```python
from build123d import *

# Parameters (mm, degrees)
SKETCH1_R               = 22.5
BOSS_EXTRUDE1_DEPTH     = 15
SKETCH2_R               = 2.75
CUT_EXTRUDE1_DEPTH      = 36.178118199
SKETCH5_R               = 8.1
CUT_EXTRUDE2_DEPTH      = 5.5
SKETCH6_R               = 5.25
CUT_EXTRUDE3_DEPTH      = 5.5
CIRPATTERN1_COUNT       = 8
SKETCH29_R              = 22.5
SKETCH29_R_2            = 12.5
CUT_EXTRUDE_THIN1_DEPTH = 2


with BuildPart() as part:
    # Sketch1 → Boss-Extrude1 (new body)
    with BuildSketch(Plane(origin=(0, 0, 0), x_dir=(0, 0, -1), z_dir=(1, 0, 0))):
        Circle(SKETCH1_R)
    extrude(amount=-BOSS_EXTRUDE1_DEPTH)

    # Sketch2 → Cut-Extrude1 (cut, through all)
    with BuildSketch(Plane(origin=(0, 0, 0), x_dir=(0, 0, -1), z_dir=(1, 0, 0))):
        Circle(SKETCH2_R)
    extrude(amount=-CUT_EXTRUDE1_DEPTH, mode=Mode.SUBTRACT)

    # Sketch5 → Cut-Extrude2 (cut)
    with BuildSketch(Plane.ZY.offset(15)):
        Circle(SKETCH5_R)
    extrude(amount=-CUT_EXTRUDE2_DEPTH, mode=Mode.SUBTRACT)

    # Sketch6 → Cut-Extrude3 (cut)
    with BuildSketch(Plane.XY.offset(22.5)):
        with Locations((-9, 0)):
            Circle(SKETCH6_R)
    cut_extrude3 = extrude(amount=-CUT_EXTRUDE3_DEPTH, mode=Mode.SUBTRACT)

    # CirPattern1: Cut-Extrude3 ×8 about axis
    cirpattern1_axis = Axis((0, 0, 0), (1, 0, 0))
    for i in range(1, CIRPATTERN1_COUNT):
        add(cut_extrude3.rotate(cirpattern1_axis, i * 360 / CIRPATTERN1_COUNT), mode=Mode.SUBTRACT)

    # Sketch29 → Cut-Extrude-Thin1 (cut)
    with BuildSketch(Plane(origin=(0, 0, 0), x_dir=(0, 0, -1), z_dir=(1, 0, 0))):
        Circle(SKETCH29_R)
        Circle(SKETCH29_R_2, mode=Mode.SUBTRACT)
    extrude(amount=-CUT_EXTRUDE_THIN1_DEPTH, mode=Mode.SUBTRACT)


solid = part.part
```
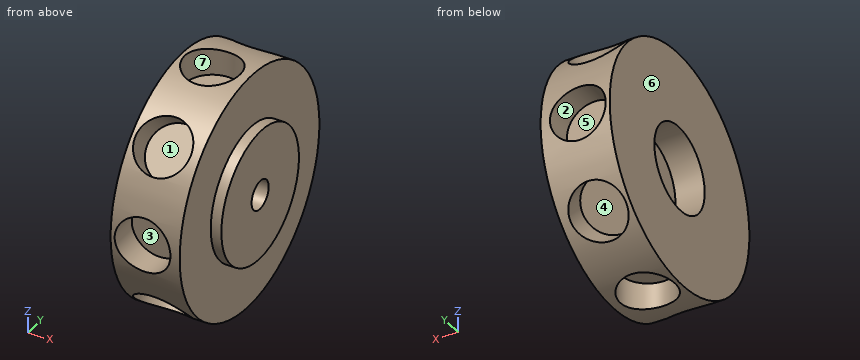
Check sheet for the modelled part. Datum: model origin and axes. Units: mm. Face numbers are marked on the shaded views. A direction names the side the tool comes from. Round coordinates to 2 decimals unless told otherwise and drop trailing zeros. Loops run counter-clockwise (first coordinate to the right, second up) from the corner with the lowest first, then second, coordinate; pieces in that order, holes last. Notation, with made-up numbers: (26.25, -21.5) -> (52.25, -21.5) arc R24 cw to (52.25, 3.5) -> close; hole circle Ø5 at (43.25, 43). An arc over 180 degrees is marked (long way). Write item = value, one per line. Start each with the question number.
1) Release check for a two-part mould opening along Y. For the marked faces 4, 5, 6 and 7 record: released by +Y, released by -Y, zero draft, split by the parting line, or undercut.
2) Sectioned sample at D-D, the plane y = 6.5. Record the cut outline in (x, z), plus the area to 3 significant figures.
3) Sectioned sample at A-A, the plane z = 0. Record the cut outline in (x, y), plus the area to 3 significant figures.
4) Set-up check for the marked faces 1, 2 and 3: record each of +Z, -Z, +X, -X, +Y, -Y from which the full face is reachable in a straight line by a thin tool's end or side.
5) Gauge pin test, flat ends, axial feed: pin 1 Ø5 at (x, y) = (-10, 1) entering from +Z; pin 2 Ø1 at (y, z) = (17, 3) entering from +X; pin 3 Ø5 at (x, y) = (-11.5, -14.5) entering from -Z. Record the tip position at first contact, or that the pin passes through.
6) Thickness scan on probe 1 along Z at (x, y) = (-6.5, -11.5); probe 2 along X at (y, z) = (0, -20); probe 3 along Y at (x, z) = (-5.25, 0). Record the ranges inside material, lowest first.
Results are:
q1.face_4 = undercut
q1.face_5 = released by +Y
q1.face_6 = zero draft
q1.face_7 = undercut
q2.outline = (-15, -21.54) -> (-2, -21.54) -> (-2, -10.68) -> (0, -10.68) -> (0, 10.68) -> (-2, 10.68) -> (-2, 21.54) -> (-15, 21.54) -> (-15, 4.83) -> (-9.5, 4.83) -> (-9.5, -4.83) -> (-15, -4.83) -> close
q2.area = 550 mm^2
q3.outline = (-15, -22.5) -> (-14.25, -22.5) -> (-14.25, -17) -> (-3.75, -17) -> (-3.75, -22.5) -> (-2, -22.5) -> (-2, -12.5) -> (0, -12.5) -> (0, -2.75) -> (-9.5, -2.75) -> (-9.5, -8.1) -> (-15, -8.1) -> close; (-15, 8.1) -> (-9.5, 8.1) -> (-9.5, 2.75) -> (0, 2.75) -> (0, 12.5) -> (-2, 12.5) -> (-2, 22.5) -> (-3.75, 22.5) -> (-3.75, 17) -> (-14.25, 17) -> (-14.25, 22.5) -> (-15, 22.5) -> close
q3.area = 378 mm^2
q4.face_1 = none
q4.face_2 = +Y
q4.face_3 = -Y
q5.pin_1 = 17
q5.pin_2 = -2
q5.pin_3 = -19.03
q6.probe_1 = -19.34 to -18.03, -12.54 to 12.54, 18.03 to 19.34
q6.probe_2 = -15 to -14.25, -3.75 to -2
q6.probe_3 = -17 to -2.75, 2.75 to 17
